Build history of the part. All positions in model axes, mm. Round coordinates to 2 decimals unless told otherwise and drop trailing zeros. Write each loop counter-clockwise with the first axis right and the second up, starting at its lowest first coordinate (ties: lowest second). Pieces come first, ordered by that corner, then holes. Notation, with made-up numbers: M 73,45 L 121,45 A17 cw 121,57 Z; hole C 27.25,-31.5 d11. An arc over 180 degrees is marked long. Use a Markdown table: item, result.
from build123d import *

# Parameters (mm, degrees)
SKETCH1_R           = 5
SKETCH1_R_2         = 22.5
SKETCH1_R_3         = 15
SKETCH1_R_4         = 7.5
BOSS_EXTRUDE1_DEPTH = 3
SKETCH3_W           = 90.5
SKETCH3_H           = 58
SKETCH3_W_2         = 77.5
SKETCH3_H_2         = 45
BOSS_EXTRUDE2_DEPTH = 3
SKETCH2_R           = 1.5
SKETCH2_R_2         = 2
CUT_EXTRUDE1_DEPTH  = 3


with BuildPart() as part:
    # Sketch1 → Boss-Extrude1 (new body)
    # profile 1 of 12: a face of its own
    with BuildSketch(Plane(origin=(0, 0, 0), x_dir=(1, 0, 0), z_dir=(0, 1, 0))):
        with BuildLine():
            Line((25, 22.5), (-30, 22.5))
            ThreePointArc((-30, 22.5), (-18.572778714, 19.382172574), (-10.3125, 10.892765661))
            ThreePointArc((-10.3125, 10.892765661), (5.929270613, 13.778379803), (15, 0))
            ThreePointArc((15, 0), (20, 5), (25, 0))
            Line((25, 0), (25, 22.5))
        make_face()
    # profile 2 of 12: a face of its own
    with BuildSketch(Plane(origin=(0, 0, 0), x_dir=(1, 0, 0), z_dir=(0, 1, 0))):
        with BuildLine():
            ThreePointArc((-10.3125, -10.892765661), (-18.572778714, -19.382172574), (-30, -22.5))
            Line((-30, -22.5), (25, -22.5))
            Line((25, -22.5), (25, 0))
            ThreePointArc((25, 0), (20, -5), (15, 0))
            ThreePointArc((15, 0), (5.929270613, -13.778379803), (-10.3125, -10.892765661))
        make_face()
    # profile 3 of 12: a face of its own
    with BuildSketch(Plane(origin=(0, 0, 0), x_dir=(1, 0, 0), z_dir=(0, 1, 0))):
        with BuildLine():
            Line((-30, 22.5), (-52.5, 22.5))
            Line((-52.5, 22.5), (-52.5, 6.7e-08))
            ThreePointArc((-52.5, 6.7e-08), (-45.909902553, 15.9099026), (-30, 22.5))
        make_face()
    # profile 4 of 12: a face of its own
    with BuildSketch(Plane(origin=(0, 0, 0), x_dir=(1, 0, 0), z_dir=(0, 1, 0))):
        with BuildLine():
            ThreePointArc((-30, -22.5), (-45.9099026, -15.909902553), (-52.5, 6.7e-08))
            Line((-52.5, 6.7e-08), (-52.5, -22.5))
            Line((-52.5, -22.5), (-30, -22.5))
        make_face()
    # profile 5 of 12: a face of its own
    with BuildSketch(Plane(origin=(0, 0, 0), x_dir=(1, 0, 0), z_dir=(0, 1, 0))):
        with Locations((20, 0)):
            Circle(SKETCH1_R)
    # profile 6 of 12: a face of its own
    with BuildSketch(Plane(origin=(0, 0, 0), x_dir=(1, 0, 0), z_dir=(0, 1, 0))):
        with Locations((-30, 0)):
            Circle(SKETCH1_R_2)
    # profile 7 of 12: a face of its own
    with BuildSketch(Plane(origin=(0, 0, 0), x_dir=(1, 0, 0), z_dir=(0, 1, 0))):
        Circle(SKETCH1_R_3)
        Circle(SKETCH1_R_4, mode=Mode.SUBTRACT)
    # profile 8 of 12: a face of its own
    with BuildSketch(Plane(origin=(0, 0, 0), x_dir=(1, 0, 0), z_dir=(0, 1, 0))):
        Circle(SKETCH1_R_4)
    # profile 9 of 12: a face of its own
    with BuildSketch(Plane(origin=(0, 0, 0), x_dir=(1, 0, 0), z_dir=(0, 1, 0))):
        Circle(SKETCH1_R_3)
    # profile 10 of 12: a face of its own
    with BuildSketch(Plane(origin=(0, 0, 0), x_dir=(1, 0, 0), z_dir=(0, 1, 0))):
        with Locations((-30, 0)):
            Circle(SKETCH1_R_2)
    # profile 11 of 12: a face of its own
    with BuildSketch(Plane(origin=(0, 0, 0), x_dir=(1, 0, 0), z_dir=(0, 1, 0))):
        with Locations((-30, 0)):
            Circle(SKETCH1_R_2)
    # profile 12 of 12: a face of its own
    with BuildSketch(Plane(origin=(0, 0, 0), x_dir=(1, 0, 0), z_dir=(0, 1, 0))):
        Circle(SKETCH1_R_3)
    extrude(amount=BOSS_EXTRUDE1_DEPTH)

    # Sketch3 → Boss-Extrude2 (add)
    with BuildSketch(Plane(origin=(0, 3, 0), x_dir=(1, 0, 0), z_dir=(0, 1, 0))):
        with Locations((-13.75, 0)):
            Rectangle(SKETCH3_W, SKETCH3_H)
        with Locations((-13.75, 0)):
            Rectangle(SKETCH3_W_2, SKETCH3_H_2, mode=Mode.SUBTRACT)
    extrude(amount=-BOSS_EXTRUDE2_DEPTH)

    # Sketch2 → Cut-Extrude1 (cut)
    with BuildSketch(Plane(origin=(0, 3, 0), x_dir=(1, 0, 0), z_dir=(0, 1, 0))):
        with BuildLine():
            Line((-26.75, 22.5), (-26.75, 5.629165125))
            ThreePointArc((-26.75, 5.629165125), (-25.403805922, 4.596194078), (-24.370834875, 3.25))
            Line((-24.370834875, 3.25), (-5.629165125, 3.25))
            ThreePointArc((-5.629165125, 3.25), (-4.596194078, 4.596194078), (-3.25, 5.629165125))
            Line((-3.25, 5.629165125), (-3.25, 22.5))
            Line((-3.25, 22.5), (-26.75, 22.5))
        make_face()
        with BuildLine():
            Line((-5.629165125, -3.25), (-24.370834875, -3.25))
            ThreePointArc((-24.370834875, -3.25), (-25.403805922, -4.596194078), (-26.75, -5.629165125))
            Line((-26.75, -5.629165125), (-26.75, -22.5))
            Line((-26.75, -22.5), (-3.25, -22.5))
            Line((-3.25, -22.5), (-3.25, -5.629165125))
            ThreePointArc((-3.25, -5.629165125), (-4.596194078, -4.596194078), (-5.629165125, -3.25))
        make_face()
        with BuildLine():
            ThreePointArc((-48, -22.5), (-49.318019485, -19.318019485), (-52.5, -18))
            Line((-52.5, -18), (-52.5, -3.25))
            Line((-52.5, -3.25), (-35.629165125, -3.25))
            ThreePointArc((-35.629165125, -3.25), (-34.596194078, -4.596194078), (-33.25, -5.629165125))
            Line((-33.25, -5.629165125), (-33.25, -22.5))
            Line((-33.25, -22.5), (-48, -22.5))
        make_face()
        with BuildLine():
            ThreePointArc((25, 4.153311931), (19.449586247, 6.47665382), (14.370834875, 3.25))
            Line((14.370834875, 3.25), (5.629165125, 3.25))
            ThreePointArc((5.629165125, 3.25), (4.596194078, 4.596194078), (3.25, 5.629165125))
            Line((3.25, 5.629165125), (3.25, 22.5))
            Line((3.25, 22.5), (20.5, 22.5))
            ThreePointArc((20.5, 22.5), (21.818019485, 19.318019485), (25, 18))
            Line((25, 18), (25, 4.153311931))
        make_face()
        with BuildLine():
            ThreePointArc((14.370834875, -3.25), (19.449586247, -6.47665382), (25, -4.153311931))
            Line((25, -4.153311931), (25, -18))
            ThreePointArc((25, -18), (21.818019485, -19.318019485), (20.5, -22.5))
            Line((20.5, -22.5), (3.25, -22.5))
            Line((3.25, -22.5), (3.25, -5.629165125))
            ThreePointArc((3.25, -5.629165125), (4.596194078, -4.596194078), (5.629165125, -3.25))
            Line((5.629165125, -3.25), (14.370834875, -3.25))
        make_face()
        with BuildLine():
            Line((-52.5, 3.25), (-52.5, 18))
            ThreePointArc((-52.5, 18), (-49.318019485, 19.318019485), (-48, 22.5))
            Line((-48, 22.5), (-33.25, 22.5))
            Line((-33.25, 22.5), (-33.25, 5.629165125))
            ThreePointArc((-33.25, 5.629165125), (-34.596194078, 4.596194078), (-35.629165125, 3.25))
            Line((-35.629165125, 3.25), (-52.5, 3.25))
        make_face()
        with Locations(Location((-52.5, 22.5, 0), (0, 0, 270))):
            Circle(SKETCH2_R)
        with Locations(Location((-30, 0, 0), (0, 0, 90))):
            Circle(SKETCH2_R_2)
        with Locations(Location((0, 0, 0), (0, 0, 270))):
            Circle(SKETCH2_R_2)
        with Locations(Location((25, 22.5, 0), (0, 0, 90))):
            Circle(SKETCH2_R)
        with Locations(Location((20, 0, 0), (0, 0, 270))):
            Circle(SKETCH2_R_2)
        with Locations(Location((25, -22.5, 0), (0, 0, 270))):
            Circle(SKETCH2_R)
        with Locations(Location((-52.5, -22.5, 0), (0, 0, 90))):
            Circle(SKETCH2_R)
    extrude(amount=-CUT_EXTRUDE1_DEPTH, mode=Mode.SUBTRACT)


solid = part.part
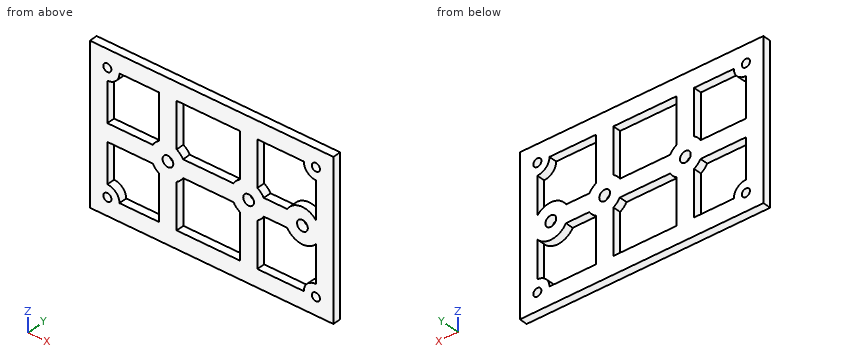
Q1. Drill centre lines: L1, parallel to X at y = 1.5, z = 0; L2, parallel to X at y = 2.2, z = -8; L3, parallel to Z at x = -41.5, y = 0.3. Where is each one in solid material? Low to high.
Response values:
| item | result |
|---|---|
| L1 | x = -59 to -32, -28 to -2, 2 to 18, 22 to 31.5 |
| L2 | x = -59 to -52.5, -33.25 to -26.75, -3.25 to 3.25, 25 to 31.5 |
| L3 | z = -29 to -22.5, -3.25 to 3.25, 22.5 to 29 |
Q2. Cut at D-D on y = 2.05. Count the separate pieces of the cut face and the enclosed holes in it, and give its area (3 significant figures).
Response values:
| item | result |
|---|---|
| separate pieces | 1 |
| enclosed holes | 13 |
| area | 2,840 mm2 |
Q3. Cut at B-B on x = -10. Give the cut face in (y, z).
Response values:
| item | result |
|---|---|
| outline | M 0,-29 L 3,-29 L 3,-22.5 L 0,-22.5 Z; M 0,-3.25 L 3,-3.25 L 3,3.25 L 0,3.25 Z; M 0,22.5 L 3,22.5 L 3,29 L 0,29 Z |
Q4. Cut at C-C on x = -30. Give the cut face in (y, z), and give its area (3 significant figures).
Response values:
| item | result |
|---|---|
| outline | M 0,-29 L 3,-29 L 3,-2 L 0,-2 Z; M 0,2 L 3,2 L 3,29 L 0,29 Z |
| area | 162 mm2 |
Q5. Cut at A-A on z = 0. Give the cut face in (x, y), and give its area (4 significant figures).
Response values:
| item | result |
|---|---|
| outline | M -59,0 L -32,0 L -32,3 L -59,3 Z; M -28,0 L -2,0 L -2,3 L -28,3 Z; M 2,0 L 18,0 L 18,3 L 2,3 Z; M 22,0 L 31.5,0 L 31.5,3 L 22,3 Z |
| area | 235.5 mm2 |
